Can you work these out from the model? Positions are in its coordinate system, mm. Round coordinates to 2 decimals unless told otherwise and drop trailing zeros. Loops run counter-clockwise (first coordinate to the right, second up) from the corner with the lowest first, then second, coordinate; pieces in that order, holes last.
(1) Will these pins go through, and if not, where does the flat tip stop? pin 1 Ø12 at (x, y) = (4.5, 7) entering from -Z (3 decimals); pin 2 Ø10 at (x, y) = (-2, 1.5) entering from +Z; pin 3 Ø5 at (x, y) = (5.5, 7.5) entering from -Z.
(2) If I drill on line 1 along Z through (x, y) = (-7.5, 2.5); line 2 along Z through (x, y) = (8.5, -9); line 3 along Y through (x, z) = (-9, -8), over which ranges is the centre line in solid material (lowest first)?
(3) I want a section at A-A on x = 4.5. Write out the boundary of the cut face in (y, z), plus the area to 3 significant figures.
(4) I want a section at C-C on y = 16.5. Write out the boundary of the cut face in (x, z).
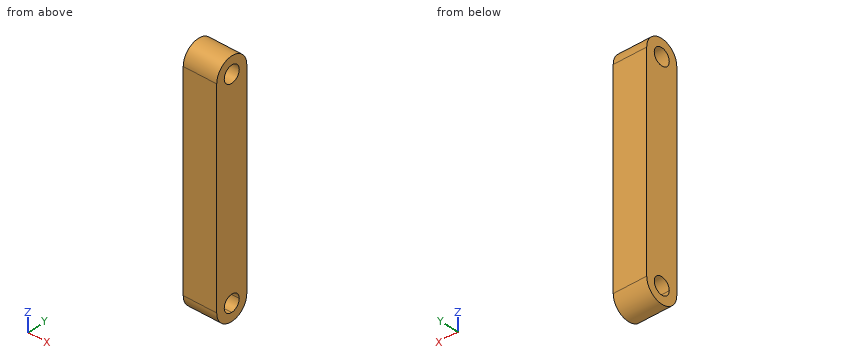
from build123d import *
from build123d.topology import SkipClean

# Parameters (mm, degrees)
BOSS_EXTRUDE1_DEPTH = 20


with BuildPart() as part:
    # Sketch1 → Boss-Extrude1 (new, symmetric)
    with SkipClean():  # the faces are left unmerged after this step: merging them gives an invalid solid
        with BuildSketch(Plane(origin=(0, 0, 0), x_dir=(0, 0, -1), z_dir=(1, 0, 0))):
            with BuildLine():
                ThreePointArc((0, 20), (-20, 0), (0, -20))
                Line((0, -20), (0, -10))
                ThreePointArc((0, -10), (-10, 0), (0, 10))
                Line((0, 10), (0, 20))
            make_face()
            with BuildLine():
                Line((0, -10), (0, -20))
                ThreePointArc((0, -20), (14.142135624, -14.142135624), (20, 0))
                ThreePointArc((20, 0), (14.142135624, 14.142135624), (0, 20))
                Line((0, 20), (0, 10))
                ThreePointArc((0, 10), (7.071067812, 7.071067812), (10, 0))
                ThreePointArc((10, 0), (7.071067812, -7.071067812), (0, -10))
            make_face()
            with BuildLine():
                ThreePointArc((20, 0), (14.142135624, -14.142135624), (0, -20))
                Line((0, -20), (250, -20))
                ThreePointArc((250, -20), (230, 0), (250, 20))
                Line((250, 20), (0, 20))
                ThreePointArc((0, 20), (14.142135624, 14.142135624), (20, 0))
            make_face()
            with BuildLine():
                ThreePointArc((250, 20), (230, 0), (250, -20))
                Line((250, -20), (250, -10))
                ThreePointArc((250, -10), (240, 0), (250, 10))
                Line((250, 10), (250, 20))
            make_face()
            with BuildLine():
                Line((250, -10), (250, -20))
                ThreePointArc((250, -20), (264.142135624, -14.142135624), (270, 0))
                ThreePointArc((270, 0), (264.142135624, 14.142135624), (250, 20))
                Line((250, 20), (250, 10))
                ThreePointArc((250, 10), (257.071067812, 7.071067812), (260, 0))
                ThreePointArc((260, 0), (257.071067812, -7.071067812), (250, -10))
            make_face()
        extrude(amount=BOSS_EXTRUDE1_DEPTH, both=True)


solid = part.part
Filled sheet:
1. pin 1: stops at z = -269.975
1. pin 2: stops at z = 20
1. pin 3: stops at z = -269.36
2. line 1: z = -269.84 to -259.68, -240.32 to -9.68, 9.68 to 19.84
2. line 2: z = -267.86 to -254.36, -245.64 to -4.36, 4.36 to 17.86
2. line 3: y = -20 to -6, 6 to 20
3. outline: (-20, -250) arc R20 ccw to (20, -250) - (20, 0) arc R20 ccw to (-20, 0) - close; hole circle Ø20 at (0, -250); hole circle Ø20 at (0, 0)
3. area: 10,600 mm2
4. outline: (-20, -261.3) - (20, -261.3) - (20, 11.3) - (-20, 11.3) - close
